Study the drawing (mm; zero at the part's minimum x, y, z) and answer. A direction names the side the tool comes from. Coordinates: 2 decimals unless noted, no trailing zeros. Order: outer loops, then holes, each group sorted by start corner. A loop starts at its lowest first (then second) coordinate and runs counter-clockwise, first axis right, second up.
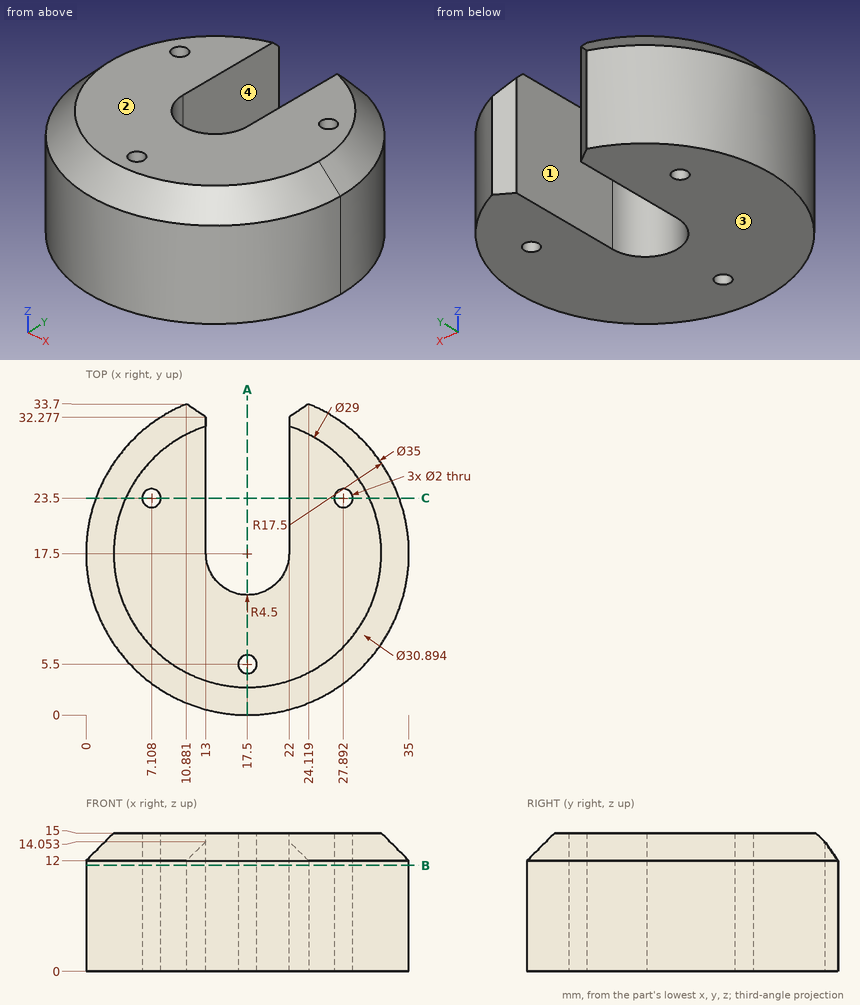
1) Straight lines are drawn through the part: line 1 (Y direction, x = 17.5, z = 2.25); line 2 (X direction, y = 18, z = 11.5); line 3 (X direction, y = 30.5, z = 8.75) (1 decimal). For each, find the intervals that lie inside material, in ascending order.
A:
line 1: y = 0 to 4.5, 6.5 to 13
line 2: x = 0.01 to 13, 22 to 34.99
line 3: x = 5.8 to 13, 22 to 29.2
2) Flat-ended cylindrical pins translate along their axes: pin 1 Ø4 at (y, z) = (3.5, 11) entering from -X; pin 2 Ø1.5 at (y, z) = (13, 4.5) entering from -X; pin 3 Ø1.5 at (x, z) = (3.5, 4.5) entering from +Y. Find the tip coordinate at first contact, or state that the pin passes through.
A:
pin 1: stops at x = 4.76
pin 2: stops at x = 0.41
pin 3: stops at y = 28.93
3) Which of the six approach directions +Z, -Z, +X, -X, +Y, -Y give full straight-line access (tool end or side, diameter ignored) to the marked faces 1 and 2?
A:
face 1: +Z, -Z, +Y
face 2: +Z, +X, -X, +Y, -Y
4) Determine the mould class of the marked faces 3 and 4 for opening direction X: pulls with the +X half, pulls with the -X half, needs draft (parallel to the pull), parting line crosses it, or undercut.
A:
face 3: needs draft
face 4: undercut
5) A cutting plane is placed at C-C, the plane y = 23.5. State how many separate pieces and enclosed holes the cut face has.
A:
separate pieces: 4
enclosed holes: 0
6) A cutting plane is placed at A-A, the plane x = 17.5. Determine the outline of the cut face in (y, z).
A:
outline: (0, 0) - (4.5, 0) - (4.5, 15) - (3, 15) - (0, 12) - close; (6.5, 0) - (13, 0) - (13, 15) - (6.5, 15) - close
7) A cutting plane is placed at B-B, the plane z = 11.5. Determine the outline of the cut face in (x, y).
A:
outline: (10.88, 33.7) arc R17.5 ccw (long way) to (24.12, 33.7) - (22, 32.28) - (22, 17.5) arc R4.5 cw to (13, 17.5) - (13, 32.28) - close; hole circle Ø2 at (7.11, 23.5); hole circle Ø2 at (17.5, 5.5); hole circle Ø2 at (27.89, 23.5)
